Verification items for the finished model (mm, model axes). Coordinates: 2 decimals unless noted, no trailing zeros. Loops run counter-clockwise (first coordinate to the right, second up) from the corner with the lowest first, then second, coordinate; pieces in that order, holes last.
Q1. Go/stop test with flat-tipped pins: P1, Ø1, axis at x = -8.5, z = 1, coming from the +Y side; P2, Ø4.5, axis at x = 0.44, y = 42.64, coming from the +Z side. Record where each tip stops, or that it passes through.
Q2. Mould release check, pull along Y, two halves, no side actions. Record for faces 1 (the face through (0, 1, 2)), 2 (the face through (0.29, -44.02, 0.92)), 3 (the face through (-0.48, -40.57, 0.77)): +Y half, -Y half, draft (parallel to the pull), parting line (faces both ways), or undercut.
Q3. Sectioned sample at B-B (z = 0.8). Enter the section's corners in (x, y).
Q4. Sectioned sample at A-A (x = 0). Enter the section's corners in (y, z), then the cut area to 3 significant figures.
Q5. Material ranges on probe 1 along Y at (x, z) = (-1, 0.15); probe 2 along Z at (x, y) = (-15.5, -39.5); probe 3 along Y at (x, z) = (0, 0.25), recorded low to high.
Q6. Sectioned sample at C-C (y = 5.5). Enter the section's corners in (x, z), then the cut area to 4 significant figures.
Q7. Sectioned sample at D-D (x = -18). Enter the section's corners in (y, z), then the cut area to 3 significant figures.
```python
from build123d import *

# Parameters (mm, degrees)
SKETCH1_W           = 42
SKETCH1_H           = 91
BOSS_EXTRUDE1_DEPTH = 2
SKETCH2_R           = 1.492291875
SKETCH2_R_2         = 1.71386304
CUT_EXTRUDE1_DEPTH  = 2
FILLET1_R           = 10


with BuildPart() as part:
    # Sketch1 → Boss-Extrude1 (new body)
    with BuildSketch(Plane.XY):
        Rectangle(SKETCH1_W, SKETCH1_H)
    extrude(amount=BOSS_EXTRUDE1_DEPTH)

    # Sketch2 → Cut-Extrude1 (cut)
    with BuildSketch(Plane.XY.offset(2)):
        with Locations((-0.283052716, -42.049438223)):
            Circle(SKETCH2_R)
        with Locations((0.438366209, 42.637044582)):
            Circle(SKETCH2_R_2)
    extrude(amount=-CUT_EXTRUDE1_DEPTH, mode=Mode.SUBTRACT)

    # Fillet1
    # the kernel refuses this fillet: 10 mm, written as the material it takes off along each edge
    with BuildSketch(Plane(origin=(-36, 45.5, 2), x_dir=(0, 0, -1), z_dir=(1, 0, 0))) as fillet1_piece_1:
        with BuildLine():
            CenterArc((10, -6), FILLET1_R, 143.130102354, 36.869897646)
            Line((0, -6), (-0.2, -6))
            Line((-0.2, -6), (-0.2, 0))
            Line((-0.2, 0), (0, 0.2))
            ThreePointArc((0, 0.2), (1, 0.2), (1.84, 0.12))
            Line((1.84, 0.12), (2, 0))
        make_face()
    extrude(amount=72, mode=Mode.SUBTRACT)
    with BuildSketch(Plane(origin=(-21, -60.5, 2), x_dir=(0, 0, -1), z_dir=(0, 1, 0)), Plane(origin=(21, 60.5, 2), x_dir=(0, 0, -1), z_dir=(0, -1, 0))) as fillet1_piece_2:
        with BuildLine():
            CenterArc((10, -6), FILLET1_R, 143.130102354, 36.869897646)
            Line((0, -6), (-0.2, -6))
            Line((-0.2, -6), (-0.2, 0))
            Line((-0.2, 0), (0, 0.2))
            ThreePointArc((0, 0.2), (1, 0.2), (1.84, 0.12))
            Line((1.84, 0.12), (2, 0))
        make_face()
    extrude(amount=121, mode=Mode.SUBTRACT)
    with BuildSketch(Plane(origin=(36, -45.5, 2), x_dir=(0, 1, 0), z_dir=(-1, 0, 0))) as fillet1_piece_3:
        with BuildLine():
            CenterArc((6, 10), FILLET1_R, 233.130102354, 36.869897646)
            Line((0, 2), (-0.12, 1.84))
            ThreePointArc((-0.12, 1.84), (-0.2, 1), (-0.2, 0))
            Line((-0.2, 0), (0, -0.2))
            Line((0, -0.2), (6, -0.2))
            Line((6, -0.2), (6, 0))
        make_face()
    extrude(amount=72, mode=Mode.SUBTRACT)


solid = part.part
```
Geometry check:
1. P1: stops at y = 44.77
1. P2: stops at z = 1.96
2. face 1: draft
2. face 2: -Y half
2. face 3: undercut
3. outline: (-19.75, -44.25) - (19.75, -44.25) - (19.75, 44.25) - (1.02, 44.25) arc R1.71 cw (long way) to (-0.14, 44.25) - (-19.75, 44.25) - close; hole circle Ø2.98 at (-0.28, -42.05)
4. outline: (-45.5, 0) - (-43.51, 0) - (-43.51, 1.16) arc R10 ccw to start; (-40.58, 0) - (40.98, 0) - (40.98, 1.89) arc R10 ccw to (39.5, 2) - (-39.5, 2) arc R10 ccw to (-40.58, 1.94) - close; (44.29, 0) - (45.5, 0) arc R10 ccw to (44.29, 0.78) - close
4. area: 165 mm2
5. probe 1: y = -45.29 to -43.36, -40.74 to 41.71, 43.57 to 45.29
5. probe 2: z = 0 to 1.99
5. probe 3: y = -45.15 to -43.51, -40.58 to 40.98, 44.29 to 45.15
6. outline: (-21, 0) - (21, 0) arc R10 ccw to (15, 2) - (-15, 2) arc R10 ccw to start
6. area: 76.35 mm2
7. outline: (-45.5, 0) - (45.5, 0) arc R10 ccw to (42.5, 1.54) - (-42.5, 1.54) arc R10 ccw to start
7. area: 136 mm2
